Source: CAD feature listing. Evaluate the final solid. Frame: model axes, mm. A direction names the side the tool comes from. Give positions to 0.01 mm unless a question says otherwise; leave off trailing zeros. Order: outer loops, then holes, each group sorted by start corner. A loop starts at its lowest first (then second) coordinate and runs counter-clockwise, first axis right, second up. Notation, with made-up numbers: (44.5, 75) - (57.5, 75) arc R30 ccw to (57.5, 102) - close; hole circle Ø3 at (81.5, 66.5). An arc over 180 degrees is marked (long way). Write each question's results on one line, items separated by ' | '. Start each with the question number.
Item 1: Section C-C on y = 7.5. Output: boundary loops of the cut face in (x, z), and give its area (3 significant figures).
Item 2: Mould query, pull axis Y, two halves, no side actions, for faces 1 (the flat face through (-27, 22, 9)), 2 (the flat face through (-15, -39.974, 20)), 3 (the cylindrical face through (-15.2, -37.51, 32.09)). Classes: released by +Y, released by -Y, zero draft, split by the parting line, or undercut.
Item 3: Section B-B on x = -14.5. Output: boundary loops of the cut face in (y, z), and give its area (3 significant figures).
Item 4: Set-up query: faces 4 (the flat face through (-8, -34.974, 20)), 5 (the flat face through (-27, 28.026, 21)), 6 (the flat face through (-26, -12, 0)). Return all of +Z, -Z, +X, -X, +Y, -Y with unobstructed straight access to the full face (end or side cutting, diameter ignored); none if empty.
Item 5: Line query: line 1 along Y through (x, z) = (-4.25, 20); line 2 along X through (y, z) = (33.5, 10); line 3 along Y through (x, z) = (-22.25, 15.5). Output: solid intervals per line, ascending.
Item 6: Section A-A on z = 25. Output: boundary loops of the cut face in (x, y), and give its area (3 significant figures).
Item 7: Contact query for flat-ended pins moving along their axis: pin 1 Ø5 at (x, z) = (-10, 21.5) entering from +Y; pin 2 Ø3 at (x, z) = (-13.53, 10.11) entering from +Y; pin 3 Ø12 at (y, z) = (6.5, 25) entering from +X. Output: stop coordinate, or through.
Item 8: Section D-D on x = -9.25. Output: boundary loops of the cut face in (y, z).
```python
from build123d import *

# Parameters (mm, degrees)
RESSALTO_EXTRUS_O1_DEPTH                   = 40
BROCA_DE_ROSQUEAR_PARA_HELICOIDE_M31_D     = 3.5
BROCA_DE_ROSQUEAR_PARA_HELICOIDE_M31_DEPTH = 10
BROCA_DE_ROSQUEAR_PARA_HELICOIDE_M31_TIP   = 1.051506083
FILETE1_R                                  = 8
ESBO_O6_W                                  = 23
ESBO_O6_H                                  = 12
CORTE_EXTRUS_O1_DEPTH                      = 10
BROCA_DE_ROSQUEAR_PARA_HELICOIDE_M33_D     = 3.5
BROCA_DE_ROSQUEAR_PARA_HELICOIDE_M33_DEPTH = 10
BROCA_DE_ROSQUEAR_PARA_HELICOIDE_M33_TIP   = 1.051506083


with BuildPart() as part:
    # Esboço1 → Ressalto-extrusão1 (new body)
    with BuildSketch(Plane.XY):
        Polygon((-30, 40.02617801), (-30, -39.97382199), (0, -39.97382199), (0, -34.97382199), (-25, -34.97382199), (-25, 40.02617801), align=None)
    extrude(amount=RESSALTO_EXTRUS_O1_DEPTH)

    # Broca de rosquear para helicoide M31
    with Locations(Plane(origin=(0, -34.97382199, 0), x_dir=(1, 0, 0), z_dir=(0, 1, 0))):
        with Locations((-13.529029312, -32.612904954), (-13.529029312, -10.11076891)):
            Hole(BROCA_DE_ROSQUEAR_PARA_HELICOIDE_M31_D / 2, depth=BROCA_DE_ROSQUEAR_PARA_HELICOIDE_M31_DEPTH)
            with Locations((0, 0, -(BROCA_DE_ROSQUEAR_PARA_HELICOIDE_M31_DEPTH + BROCA_DE_ROSQUEAR_PARA_HELICOIDE_M31_TIP / 2))):  # 118° drill point
                Cone(0, BROCA_DE_ROSQUEAR_PARA_HELICOIDE_M31_D / 2, BROCA_DE_ROSQUEAR_PARA_HELICOIDE_M31_TIP, mode=Mode.SUBTRACT)

    # Filete1
    filete1_edges = [part.edges().sort_by_distance(p)[0] for p in [
        (-25, -34.97382199, 20),
    ]]
    fillet(filete1_edges, radius=FILETE1_R)

    # Esboço6 → Corte-extrusão1 (cut)
    with BuildSketch(Plane(origin=(-25, 0, 0), x_dir=(0, 0, -1), z_dir=(1, 0, 0))):
        with Locations((-20.5, 22.02617801)):
            Rectangle(ESBO_O6_W, ESBO_O6_H)
    extrude(amount=-CORTE_EXTRUS_O1_DEPTH, mode=Mode.SUBTRACT)

    # Broca de rosquear para helicoide M33
    with Locations(Plane(origin=(-25, 0, 0), x_dir=(0, 0, -1), z_dir=(1, 0, 0))):
        with Locations((-6.454548455, 21.588594031), (-34.28528994, 21.588594031)):
            Hole(BROCA_DE_ROSQUEAR_PARA_HELICOIDE_M33_D / 2, depth=BROCA_DE_ROSQUEAR_PARA_HELICOIDE_M33_DEPTH)
            with Locations((0, 0, -(BROCA_DE_ROSQUEAR_PARA_HELICOIDE_M33_DEPTH + BROCA_DE_ROSQUEAR_PARA_HELICOIDE_M33_TIP / 2))):  # 118° drill point
                Cone(0, BROCA_DE_ROSQUEAR_PARA_HELICOIDE_M33_D / 2, BROCA_DE_ROSQUEAR_PARA_HELICOIDE_M33_TIP, mode=Mode.SUBTRACT)


solid = part.part
```
Evaluation:
1) outline: (-30, 0) - (-25, 0) - (-25, 40) - (-30, 40) - close | area: 200 mm^2
2) face 1: undercut | face 2: released by -Y | face 3: zero draft
3) outline: (-39.97, 0) - (-34.97, 0) - (-34.97, 8.65) - (-39.97, 8.65) - close; (-39.97, 11.57) - (-34.97, 11.57) - (-34.97, 31.16) - (-39.97, 31.16) - close; (-39.97, 34.07) - (-34.97, 34.07) - (-34.97, 40) - (-39.97, 40) - close | area: 171 mm^2
4) face 4: +Z, -Z, +X, +Y | face 5: +X, -X | face 6: -Z, +X, -X, +Y, -Y
5) line 1: y = -39.97 to -34.97 | line 2: x = -30 to -25 | line 3: y = -39.97 to -33.01
6) outline: (-30, -39.97) - (0, -39.97) - (0, -34.97) - (-17, -34.97) arc R8 cw to (-25, -26.97) - (-25, 16.03) - (-30, 16.03) - close; (-30, 28.03) - (-25, 28.03) - (-25, 40.03) - (-30, 40.03) - close | area: 479 mm^2
7) pin 1: stops at y = -34.97 | pin 2: passes through | pin 3: stops at x = -25
8) outline: (-39.97, 0) - (-34.97, 0) - (-34.97, 40) - (-39.97, 40) - close
